```python
from build123d import *

# Parameters (mm, degrees)
F0_W     = 50.8
F0_H     = 50.8
F1_DEPTH = 50.8
F2_R     = 15.755005
F3_DEPTH = 50.8
F4_R     = 19.05
F5_DEPTH = 50.8


with BuildPart() as f1:
    # F0 (on Front) → F1 (new body)
    with BuildSketch(Plane.XZ):
        with Locations((25.4, 25.4)):
            Rectangle(F0_W, F0_H)
    extrude(amount=F1_DEPTH)

    # F2 (on face) → F3 (cut)
    with BuildSketch(Plane.XZ.offset(50.8)):
        with Locations((24.034012, 24.344128)):
            Circle(F2_R)
    extrude(amount=F3_DEPTH, mode=Mode.SUBTRACT)

    # F4 (on face) → F5 (cut)
    with BuildSketch(Plane.XZ.offset(50.8)):
        with Locations((25.4, 25.4)):
            Circle(F4_R)
    extrude(amount=-F5_DEPTH, mode=Mode.SUBTRACT)


solid = f1.part
```
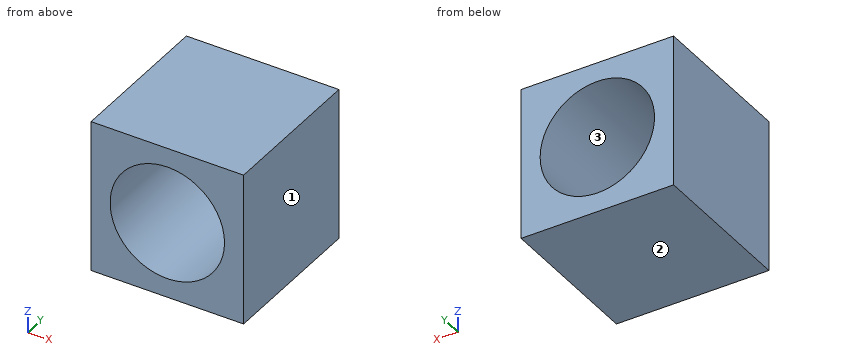
Model file for the job. Use its own axes, mm. Face numbers are marked on the shaded views. Coordinates: 2 decimals unless noted, no trailing zeros. Write each loop counter-clockwise with the first axis right and the second up, starting at its lowest first coordinate (ties: lowest second). Pieces come first, ordered by that corner, then holes. Notation, with made-up numbers: (73, 85.25) - (121, 85.25) arc R27 cw to (121, 120.25) - close; hole circle Ø5 at (-22.5, -13). An arc over 180 degrees is marked (long way). Use a Markdown table: item, result. Add a question column.
Item 1: Band-saw the part on A-A, the plane z = 25.4. Write the cut outline in (x, y), and give its area (3 significant figures).
Item 2: Drop a flat-ended pin along its axis: pin 1 (2 mm diameter, centred on y = -45, z = 23, fed in from -X). Give the stop position or say it passes through.
Item 3: Band-saw the part on C-C, the plane y = -27. Write the cut outline in (x, z), and give its area (3 significant figures).
Item 4: Band-saw the part on B-B, the plane x = 25.4. Write the cut outline in (y, z).
Item 5: Two-plate mould, pull along X, no slides. Class the marked faces 1, 2 and 3: pulls with the +X half, pulls with the -X half, needs draft (parallel to the pull), parting line crosses it, or undercut.
Item 6: Drill centre lines: line 1 along X through (y, z) = (-32.5, 25); line 2 along Z through (x, y) = (20.5, -46.5). Where is each one in solid material? Low to high.
A:
| question | item | result |
|---|---|---|
| 1 | outline | (0, -50.8) - (6.35, -50.8) - (6.35, 0) - (0, 0) - close; (44.45, -50.8) - (50.8, -50.8) - (50.8, 0) - (44.45, 0) - close |
| 1 | area | 645 mm² |
| 2 | pin 1 | stops at x = 0 |
| 3 | outline | (0, 0) - (50.8, 0) - (50.8, 50.8) - (0, 50.8) - close; hole circle Ø38.1 at (25.4, 25.4) |
| 3 | area | 1,440 mm² |
| 4 | outline | (-50.8, 0) - (0, 0) - (0, 6.35) - (-50.8, 6.35) - close; (-50.8, 44.45) - (0, 44.45) - (0, 50.8) - (-50.8, 50.8) - close |
| 5 | face 1 | pulls with the +X half |
| 5 | face 2 | needs draft |
| 5 | face 3 | undercut |
| 6 | line 1 | x = 0 to 6.35, 44.45 to 50.8 |
| 6 | line 2 | z = 0 to 6.99, 43.81 to 50.8 |
